Read the model definition and answer for the solid it produces. Units are mm, in the model's axes. Coordinates: 2 decimals unless noted, no trailing zeros. Order: outer loops, then holes, each group sorted by start corner. A loop starts at its lowest first (then second) coordinate and runs counter-clockwise, first axis right, second up. Notation, with made-up numbers: (67.25, 1.5) -> (124.25, 1.5) arc R13 cw to (124.25, 26.5) -> close; hole circle Ø1 at (84, 84). An arc over 180 degrees is marked (long way). Return JSON: item names as keys, results as strings. Group by question number.
```python
from build123d import *

# Parameters (mm, degrees)
F1_W = 19.05
F1_H = 76.2


with BuildPart() as f2:
    # F2: sweep along a path in F0
    with BuildLine(Plane.XY) as f2_path:
        Line((0, 0), (0, -590.55))
        Line((0, -590.55), (1879.6, -590.55))
    # F1 (on Front) → F2 (sweep)
    with BuildSketch(Plane.XZ):
        with Locations((-9.525, 38.1)):
            Rectangle(F1_W, F1_H)
    sweep(path=f2_path.line, transition=Transition.RIGHT)


solid = f2.part
```
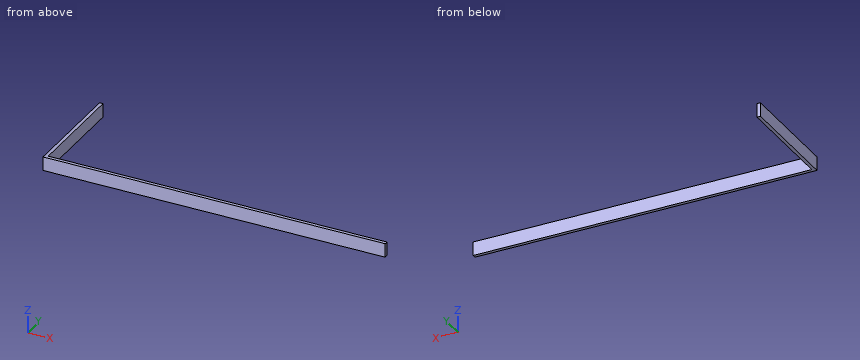
1. Find section B-B on x = 726.5. Determine the outline of the cut face in (y, z).
2. Straight lines are drawn through the part: L1, parallel to X at y = -262.5, z = 39; L2, parallel to Y at x = 1590, z = 24. For each, find the intervals that lie inside material, in ascending order.
3. Find section C-C on z = 57.5. Determine the outline of the cut face in (x, y), and give its area (3 significant figures).
4. Find section A-A on y = -203. Determine the outline of the cut face in (x, z), and give its area (3 significant figures).
Result:
{
 "1": {"outline": "(-609.6, 0) -> (-590.55, 0) -> (-590.55, 76.2) -> (-609.6, 76.2) -> close"},
 "2": {"L1": "-19.05 to 0", "L2": "-609.6 to -590.55"},
 "3": {"outline": "(-19.05, -609.6) -> (1879.6, -609.6) -> (1879.6, -590.55) -> (0, -590.55) -> (0, 0) -> (-19.05, 0) -> close", "area": "47,400 mm^2"},
 "4": {"outline": "(-19.05, 0) -> (0, 0) -> (0, 76.2) -> (-19.05, 76.2) -> close", "area": "1,450 mm^2"}
}
